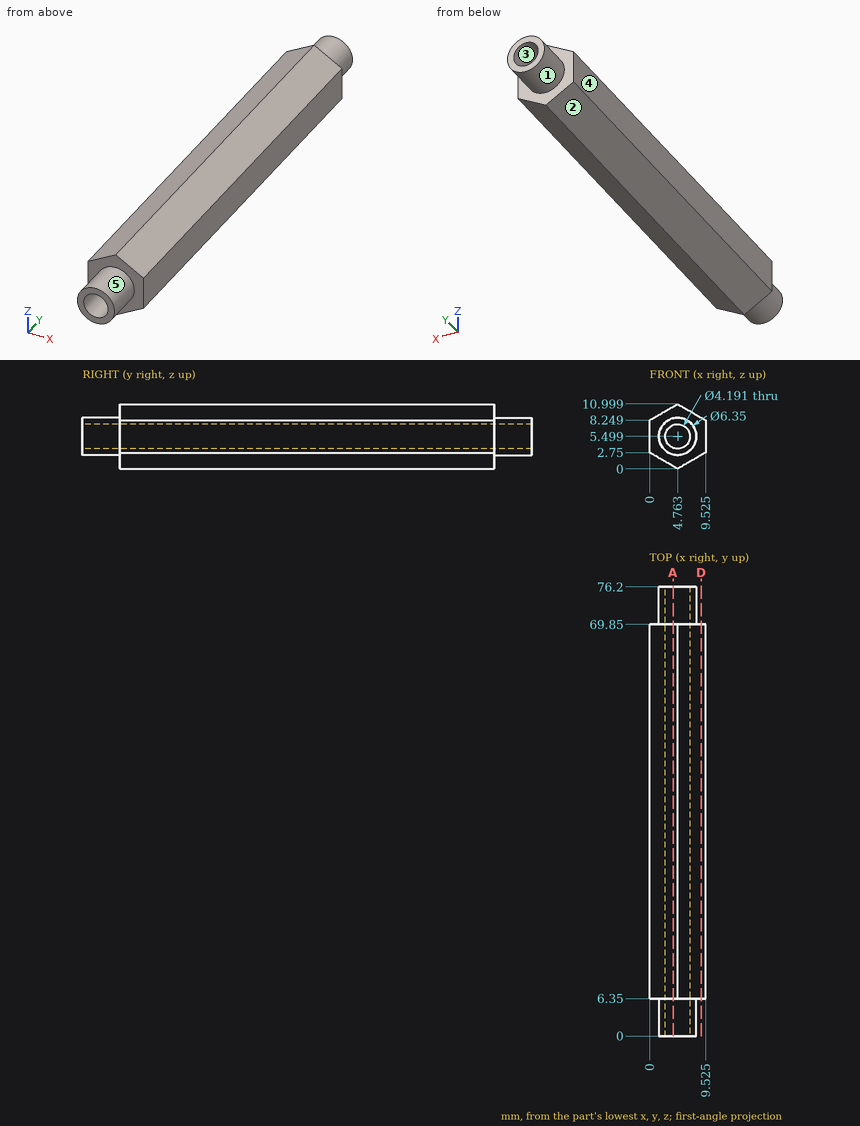
Here's the drawing with two shaded views (mm, measured from the low corner). I have some questions. A direction names the side the tool comes from. Coordinates: 2 decimals unless noted, no trailing zeros. Order: outer loops, then holes, each group sorted by start corner. A loop starts at its lowest first (then second) coordinate and runs counter-clockwise, first axis right, second up.
Item 1: If we section it at D-D on x = 8.75: List the corners of the cut face in (y, z) for me.
Result sheet:
outline: (6.35, 2.3) - (69.85, 2.3) - (69.85, 8.7) - (6.35, 8.7) - close
Item 2: If we mould it in two halves opening along X, with no side actions, what happens to the marked faces 3, 4 and 5? For each: +X half, -X half, draft (parallel to the pull), parting line (faces both ways), or undercut.
Result sheet:
face 3: undercut
face 4: -X half
face 5: parting line
Item 3: For P1, Ø3, axis at x = 3, y = 58, coming from the -Z side; P2, Ø2, axis at x = 3, y = 37, coming from the -Z side, each with a flat end and sliding along its axis, tell me the tip position at first contact or that it passes through.
Result sheet:
P1: stops at z = 0.15
P2: stops at z = 0.44
Item 4: I need wall thicknesses on line 1 (Y direction, x = 5.25, z = 2.25); line 2 (X direction, y = 15.5, z = 4) (1 decimal); line 3 (Z direction, x = 5.25, y = 10.5) (1 decimal). Which ranges of each line are inside material? Lowest first, please.
Result sheet:
line 1: y = 6.35 to 69.85
line 2: x = 0 to 3.3, 6.2 to 9.5
line 3: z = 0.3 to 3.5, 7.5 to 10.7
Item 5: For the marked faces 1 and 2, which set-ups out of +Z, -Z, +X, -X, +Y, -Y let a thin tool reach every point of the face, with its end or its side?
Result sheet:
face 1: +Y
face 2: -Z, -X, +Y, -Y
Item 6: If we section it at A-A on x = 4: List the corners of the cut face in (y, z) for me.
Result sheet:
outline: (0, 2.42) - (6.35, 2.42) - (6.35, 0.44) - (69.85, 0.44) - (69.85, 2.42) - (76.2, 2.42) - (76.2, 3.55) - (0, 3.55) - close; (0, 7.45) - (76.2, 7.45) - (76.2, 8.58) - (69.85, 8.58) - (69.85, 10.56) - (6.35, 10.56) - (6.35, 8.58) - (0, 8.58) - close
